from build123d import *

# Parameters (mm, degrees)
SKETCH1_W           = 150
SKETCH1_H           = 120
SKETCH1_R           = 1.75
BOSS_EXTRUDE1_DEPTH = 2.5


with BuildPart() as part:
    # Sketch1 → Boss-Extrude1 (new body)
    with BuildSketch(Plane(origin=(0, 0, 0), x_dir=(0, 0, -1), z_dir=(1, 0, 0))):
        Rectangle(SKETCH1_W, SKETCH1_H)
        with Locations((50, 52)):
            Circle(SKETCH1_R, mode=Mode.SUBTRACT)
        with Locations((-71, 52)):
            Circle(SKETCH1_R, mode=Mode.SUBTRACT)
        with Locations(Location((50, -52, 0), (0, 0, 180))):
            Circle(SKETCH1_R, mode=Mode.SUBTRACT)
    extrude(amount=BOSS_EXTRUDE1_DEPTH)


solid = part.part
The model under review builds one solid part; all positions refer to its coordinate system, in mm. Round coordinates to 2 decimals unless told otherwise and drop trailing zeros. Write each loop counter-clockwise with the first axis right and the second up, starting at its lowest first coordinate (ties: lowest second). Pieces come first, ordered by that corner, then holes. Notation, with made-up numbers: (65, 82.25) - (118, 82.25) arc R21 cw to (118, 97.25) - close; hole circle Ø5 at (-35.5, -36.5). An arc over 180 degrees is marked (long way). One line per item, written item: value. Start each with the question number.
1. To check wall thickness, follow L1, parallel to Y at x = 2, z = -50; L2, parallel to Y at x = 0.7, z = 71; L3, parallel to Z at x = 1.45, y = -52. State the ranges of each line that lie inside material, in increasing order. Write a range as from..to.
2. Consider section B-B on y = -52. Write out the cut boundary in (x, z), and give its area (3 significant figures).
3. Consider section A-A on z = 71. Write out the cut boundary in (x, y), and give its area (3 significant figures).
4. Consider section D-D on z = -50. Write out the cut boundary in (x, y), and give its area (4 significant figures).
5. Clearance check with a flat-ended pin moving along its axis: P1, Ø2, axis at y = 52, z = -50, coming from the -X side. State where the tip first meets the part, or that it passes through.
6. The part is to be moulded in two halves that separate along Y. For faces 1 (the face through (1.232, 51.33, 69.383)), 2 (the face through (0, 1, 1)), say which applies: released by +Y, released by -Y, zero draft, split by the parting line, or undercut.
7. Consider section C-C on y = 52. Write out the cut boundary in (x, z), and give its area (4 significant figures).
Checks:
1. L1: y = -60..-53.75, -50.25..50.25, 53.75..60
1. L2: y = -60..50.25, 53.75..60
1. L3: z = -75..-51.75, -48.25..75
2. outline: (0, -75) - (2.5, -75) - (2.5, -51.75) - (0, -51.75) - close; (0, -48.25) - (2.5, -48.25) - (2.5, 75) - (0, 75) - close
2. area: 366 mm^2
3. outline: (0, -60) - (2.5, -60) - (2.5, 50.25) - (0, 50.25) - close; (0, 53.75) - (2.5, 53.75) - (2.5, 60) - (0, 60) - close
3. area: 291 mm^2
4. outline: (0, -60) - (2.5, -60) - (2.5, -53.75) - (0, -53.75) - close; (0, -50.25) - (2.5, -50.25) - (2.5, 50.25) - (0, 50.25) - close; (0, 53.75) - (2.5, 53.75) - (2.5, 60) - (0, 60) - close
4. area: 282.5 mm^2
5. P1: passes through
6. face 1: undercut
6. face 2: zero draft
7. outline: (0, -75) - (2.5, -75) - (2.5, -51.75) - (0, -51.75) - close; (0, -48.25) - (2.5, -48.25) - (2.5, 69.25) - (0, 69.25) - close; (0, 72.75) - (2.5, 72.75) - (2.5, 75) - (0, 75) - close
7. area: 357.5 mm^2
